from build123d import *

# Parameters (mm, degrees)
SKETCH1_W                   = 25.4
SKETCH1_H                   = 19.05
BOSS_EXTRUDE1_DEPTH         = 7.112
SKETCH2_W                   = 25.4
SKETCH2_H                   = 6.35
BOSS_EXTRUDE2_DEPTH         = 5.588
F_32_0_116_DIAMETER_HOLE1_D = 2.9464


with BuildPart() as part:
    # Sketch1 → Boss-Extrude1 (new body)
    with BuildSketch(Plane(origin=(0, 0, 0), x_dir=(1, 0, 0), z_dir=(0, 1, 0))):
        with Locations((12.7, 9.525)):
            Rectangle(SKETCH1_W, SKETCH1_H)
    extrude(amount=BOSS_EXTRUDE1_DEPTH)

    # Sketch2 → Boss-Extrude2 (add)
    with BuildSketch(Plane(origin=(0, 7.112, 0), x_dir=(1, 0, 0), z_dir=(0, 1, 0))):
        with Locations((12.7, 15.875)):
            Rectangle(SKETCH2_W, SKETCH2_H)
    extrude(amount=BOSS_EXTRUDE2_DEPTH)

    # #32 (0.116) Diameter Hole1 (through all)
    with Locations(Plane(origin=(0, 7.112, 0), x_dir=(1, 0, 0), z_dir=(0, 1, 0))):
        with Locations((12.7, 6.35)):
            Hole(F_32_0_116_DIAMETER_HOLE1_D / 2)


solid = part.part
Verification items for the finished model (mm, model axes). A direction names the side the tool comes from. Give positions to 0.01 mm unless a question says otherwise; leave off trailing zeros. Loops run counter-clockwise (first coordinate to the right, second up) from the corner with the lowest first, then second, coordinate; pieces in that order, holes last. Notation, with made-up numbers: (83.25, -23.75) - (127.25, -23.75) arc R22 ccw to (127.25, -3.75) - close; hole circle Ø3 at (0.5, 17.5). An arc over 180 degrees is marked (long way). Write each question's results on one line, items separated by ' | '.
1) Mould release check, pull along X, two halves, no side actions. Record for faces 1 (the cylindrical face through (11.295, 3.506, -6.793)), 2 (the flat face through (0, 5, -12)), 3 (the flat face through (13, 4, 0)): pulls with the +X half, pulls with the -X half, needs draft (parallel to the pull), parting line crosses it, or undercut.
Solution:
face 1: undercut | face 2: pulls with the -X half | face 3: needs draft
2) Sectioned sample at D-D on x = 17.5. Record the boundary of the cut face in (y, z).
Solution:
outline: (0, -19.05) - (12.7, -19.05) - (12.7, -12.7) - (7.11, -12.7) - (7.11, 0) - (0, 0) - close
3) Depth check by flat-ended pin: P1, Ø2, axis at x = 6.5, z = -3, coming from the +Y side. Enter the tip coordinate at first touch or a pass-through.
Solution:
P1: y = 7.11
4) Sectioned sample at A-A on z = -6.35. Record the boundary of the cut face in (x, y).
Solution:
outline: (0, 0) - (11.23, 0) - (11.23, 7.11) - (0, 7.11) - close; (14.17, 0) - (25.4, 0) - (25.4, 7.11) - (14.17, 7.11) - close
5) Sectioned sample at B-B on x = 12.7. Record the boundary of the cut face in (y, z).
Solution:
outline: (0, -19.05) - (12.7, -19.05) - (12.7, -12.7) - (7.11, -12.7) - (7.11, -7.82) - (0, -7.82) - close; (0, -4.88) - (7.11, -4.88) - (7.11, 0) - (0, 0) - close
6) Tool access check on faces 4 (the flat face through (13, 10, -12.7)), 5 (the flat face through (13, 6, -19.05)). Record the directions out of +Z, -Z, +X, -X, +Y, -Y that give a thin tool (end or side, any length) a straight path to the whole face; none if there is none.
Solution:
face 4: +Z, +X, -X, +Y | face 5: -Z, +X, -X, +Y, -Y
7) Sectioned sample at C-C on y = 9.25. Record the boundary of the cut face in (x, z).
Solution:
outline: (0, -19.05) - (25.4, -19.05) - (25.4, -12.7) - (0, -12.7) - close
8) Material ranges on L1, parallel to Z at x = 12.7, y = 3; L2, parallel to X at y = 5.25, z = -6.35; L3, parallel to Y at x = 16.5, z = -12.25, recorded low to high. Write a range as from..to.
Solution:
L1: -19.05..-7.82, -4.88..0 | L2: 0..11.23, 14.17..25.4 | L3: 0..7.11
